Part model, mm, in its own coordinate system. Round coordinates to 2 decimals unless told otherwise and drop trailing zeros. Order: outer loops, then holes, each group sorted by start corner. A loop starts at its lowest first (then second) coordinate and runs counter-clockwise, first axis right, second up. Notation, with made-up numbers: (63.5, 11) -> (82.5, 11) arc R10 cw to (82.5, 20) -> close; hole circle Ø8 at (23, 24.5). An arc over 180 degrees is marked (long way). Return JSON: item names as keys, results as strings. Group by question number.
Autodesk Inventor part; units mm, degrees
ref_plane "YZ Plane" through (0, 0, 0) normal (1, 0, 0) x (0, 1, 0)
ref_plane "XZ Plane" through (0, 0, 0) normal (0, 1, 0) x (-1, 0, 0)
ref_plane "XY Plane" through (0, 0, 0) normal (0, 0, 1) x (1, 0, 0)
sketch "Sketch1" plane through (0, 0, 0) normal (0, 0, 1) x (1, 0, 0)
  circle A0 centre (0, 0) radius 32.385
  circle A1 centre (-48.4934, 48.4934) radius 32.385
  circle A2 centre (48.4934, 48.4934) radius 32.385
  circle A3 centre (0, 0) radius 68.58 construction
  line L0 (-48.4934, 48.4934) -> (48.4934, 48.4934) construction
  circle A4 centre (-48.4934, -48.4934) radius 32.385 construction
  circle A5 centre (48.4934, -48.4934) radius 32.385 construction
  line L1 (-48.4934, 48.4934) -> (-48.4934, -48.4934) construction
  circle A6 centre (0, 0) radius 36.195
  circle A7 centre (-48.4934, 48.4934) radius 36.195
  circle A8 centre (48.4934, 48.4934) radius 36.195
  arc A9 (-24.2467, 75.3667) -> (24.2467, 75.3667) centre (0, 102.24) ccw
  arc A10 (-34.6636, -10.4169) -> (-58.9103, 13.8298) centre (-69.3272, -20.8338) ccw
  arc A11 (58.9103, 13.8298) -> (34.6636, -10.4169) centre (69.3272, -20.8338) ccw
  dimension "d0" = 137.16
  dimension "d1" = 64.77
extrude "Extrusion1" add sketch "Sketch1" along normal blind 6.35 contours A0 A8 A6 A7 | A0 A7 A6 A8 | A8 A6 | A7 A6 | A8 A6 | A6 A7 A9 A8 | A8 A11 A6 | A7 A6 | A6 A10 A7
properties part number "Flywheel Gearbox Holder"
(1) Probe L1, parallel to Y at x = 0, z = 4 (3 decimals); L2, parallel to X at y = 26.5, z = 0.5; L3, parallel to X at y = 22.5, z = 0.5. List the from-to ranges inside material, lowest first. Write a range as [from, to].
(2) Saw through at D-D, the plane y = 55. List the corners of the cut face in (x, z), and give its area (3 significant figures).
(3) Saw through at B-B, the plane y = -2. List the corners of the cut face in (x, z), and give its area (3 significant figures).
(4) Pin check, flat tips, straight feed: P1, Ø3, axis at y = 25, z = 4.5, coming from the -X side; P2, Ø1.5, axis at y = 72, z = 2, coming from the +X side; P3, Ø2, axis at x = 8, z = 1, coming from the -Y side. Stop position of each tip, or through.
(5) Mould opens along X. For faces 1 (the cylindrical face through (0.65, -36.19, 3.13)), 2 (the cylindrical face through (-43.911, 4.936, 3.131)), 3 (the cylindrical face through (-80.465, 65.461, 3.131)) say: pulls with the +X half, pulls with the -X half, needs draft (parallel to the pull), parting line crosses it, or undercut.
(6) Saw through at C-C, the plane z = 5. List the corners of the cut face in (x, y) (3 decimals), and give its area (3 significant figures).
(7) Saw through at A-A, the plane x = 0. List the corners of the cut face in (y, z) (3 decimals), and give its area (3 significant figures).
Results are:
{
 "1": {"L1": "y = [-36.195, -32.385], [32.385, 66.045]", "L2": "x = [-77.24, -72.26], [-24.72, -18.62], [18.62, 24.72], [72.26, 77.24]", "L3": "x = [-73.68, -67.81], [-29.18, -23.29], [23.29, 29.18], [67.81, 73.68]"},
 "2": {"outline": "(-84.1, 0) -> (-80.22, 0) -> (-80.22, 6.35) -> (-84.1, 6.35) -> close; (-16.77, 0) -> (16.77, 0) -> (16.77, 6.35) -> (-16.77, 6.35) -> close; (80.22, 0) -> (84.1, 0) -> (84.1, 6.35) -> (80.22, 6.35) -> close", "area": "262 mm^2"},
 "3": {"outline": "(-38.42, 0) -> (-32.32, 0) -> (-32.32, 6.35) -> (-38.42, 6.35) -> close; (32.32, 0) -> (38.42, 0) -> (38.42, 6.35) -> (32.32, 6.35) -> close", "area": "77.4 mm^2"},
 "4": {"P1": "stops at x = -77.24", "P2": "stops at x = 76.64", "P3": "stops at y = -35.51"},
 "5": {"face 1": "parting line crosses it", "face 2": "pulls with the -X half", "face 3": "undercut"},
 "6": {"outline": "(-58.91, 13.83) arc R36.195 cw to (-34.664, -10.417) arc R36.195 ccw to (34.664, -10.417) arc R36.195 cw to (58.91, 13.83) arc R36.195 ccw (long way) to (24.247, 75.367) arc R36.195 cw to (-24.247, 75.367) arc R36.195 ccw (long way) to start; hole circle Ø64.77 at (-48.493, 48.493); hole circle Ø64.77 at (0, 0); hole circle Ø64.77 at (48.493, 48.493)", "area": "3,560 mm^2"},
 "7": {"outline": "(-36.195, 0) -> (-32.385, 0) -> (-32.385, 6.35) -> (-36.195, 6.35) -> close; (32.385, 0) -> (66.045, 0) -> (66.045, 6.35) -> (32.385, 6.35) -> close", "area": "238 mm^2"}
}
